For this review, take the finished solid that the model builds, in its own axes (mm). A direction names the side the tool comes from. Coordinates: 2 decimals unless noted, no trailing zeros. Order: outer loops, then holes, each group sorted by start corner. A loop starts at its lowest first (then second) coordinate and runs counter-clockwise, first axis right, second up.
from build123d import *

# Parameters (mm, degrees)
ESQUISSE1_W          = 50
ESQUISSE1_H          = 30
BASE_EXTRUSION_DEPTH = 10
PER_AGE1_D           = 5
PER_AGE1_CSINK_D     = 11
PER_AGE1_CSINK_ANGLE = 90
PER_AGE2_D           = 6
PER_AGE2_CBORE_D     = 11
PER_AGE2_CBORE_DEPTH = 6
CHANFREIN1_SIZE      = 5


with BuildPart() as part:
    # Esquisse1 → Base-Extrusion (new body)
    with BuildSketch(Plane.XY):
        with Locations((0, 15)):
            Rectangle(ESQUISSE1_W, ESQUISSE1_H)
    extrude(amount=BASE_EXTRUSION_DEPTH)

    # Perçage1 (through all)
    with Locations(Plane.XY.offset(10)):
        with Locations((15, 7.5)):
            per_age1 = CounterSinkHole(PER_AGE1_D / 2, PER_AGE1_CSINK_D / 2, counter_sink_angle=PER_AGE1_CSINK_ANGLE)

    # Symétrie1: Perçage1 across plane
    add(per_age1.mirror(Plane(origin=(0, 0, 0), x_dir=(0, 0, 1), z_dir=(1, 0, 0))), mode=Mode.SUBTRACT)

    # Perçage2 (through all)
    with Locations(Plane(origin=(0, 0, 0), x_dir=(-1, 0, 0), z_dir=(0, 0, -1))):
        with Locations((-15, 22.5)):
            per_age2 = CounterBoreHole(PER_AGE2_D / 2, PER_AGE2_CBORE_D / 2, PER_AGE2_CBORE_DEPTH)

    # Symétrie2: Perçage2 across plane
    add(per_age2.mirror(Plane(origin=(0, 0, 0), x_dir=(0, 0, 1), z_dir=(1, 0, 0))), mode=Mode.SUBTRACT)

    # Chanfrein1
    chanfrein1_edges = [part.edges().sort_by_distance(p)[0] for p in [
        (-25, 0, 5),
        (25, 0, 5),
    ]]
    chamfer(chanfrein1_edges, length=CHANFREIN1_SIZE)


solid = part.part
1. Take a section at A-A, the plane y = 7.5. Give the boundary of the cut face in (x, z).
Answer below:
outline: (-25, 0) - (-17.5, 0) - (-17.5, 7) - (-20.5, 10) - (-25, 10) - close; (-12.5, 0) - (12.5, 0) - (12.5, 7) - (9.5, 10) - (-9.5, 10) - (-12.5, 7) - close; (17.5, 0) - (25, 0) - (25, 10) - (20.5, 10) - (17.5, 7) - close
2. To check wall thickness, follow L1, parallel to Y at x = 15, z = 3.5; L2, parallel to X at y = 7.5, z = 4; L3, parallel to Y at x = -14, z = 8.5. State the ranges of each line that lie inside material, in increasing order.
Answer below:
L1: y = 0 to 5, 10 to 17, 28 to 30
L2: x = -25 to -17.5, -12.5 to 12.5, 17.5 to 25
L3: y = 0 to 3.63, 11.37 to 19.67, 25.33 to 30
3. Take a section at B-B, the plane x = -15. Give the boundary of the cut face in (y, z).
Answer below:
outline: (0, 0) - (5, 0) - (5, 7) - (2, 10) - (0, 10) - close; (10, 0) - (17, 0) - (17, 6) - (19.5, 6) - (19.5, 10) - (13, 10) - (10, 7) - close; (25.5, 6) - (28, 6) - (28, 0) - (30, 0) - (30, 10) - (25.5, 10) - close
4. Machinability: for faces 1 (the face through (-12, 22.6, 8)), 2 (the face through (15.716, 27.953, 2.958)), which of the approach directions +Z, -Z, +X, -X, +Y, -Y give a long, thin tool a straight path to every point of the face, cutting with its end or side? Answer none if there is none.
Answer below:
face 1: +Z, -Z
face 2: -Z
5. Clearance check with flat-ended pins moving along their axes: pin 1 Ø3.5 at (x, y) = (-15, 22.5) entering from -Z; pin 2 Ø8 at (x, y) = (15, 22.5) entering from -Z. State where each tip first meets the part, or that it passes through.
Answer below:
pin 1: passes through
pin 2: stops at z = 6
6. Take a section at C-C, the plane y = 22.5. Give the boundary of the cut face in (x, z), plus the area to 3 significant figures.
Answer below:
outline: (-25, 0) - (-20.5, 0) - (-20.5, 6) - (-18, 6) - (-18, 10) - (-25, 10) - close; (-12, 6) - (-9.5, 6) - (-9.5, 0) - (9.5, 0) - (9.5, 6) - (12, 6) - (12, 10) - (-12, 10) - close; (18, 6) - (20.5, 6) - (20.5, 0) - (25, 0) - (25, 10) - (18, 10) - close
area: 320 mm2
7. Take a section at D-D, the plane x = 16. Give the number of separate pieces and of enclosed holes in the cut face, plus the area to 3 significant figures.
Answer below:
separate pieces: 3
enclosed holes: 0
area: 157 mm2
8. The part is to be moulded in two halves that separate along X. For faces 3 (the face through (-25, 17, 5)), 4 (the face through (-13, 20, 6)), 5 (the face through (23, 3, 5)), say which applies: +X half, -X half, draft (parallel to the pull), parting line (faces both ways), or undercut.
Answer below:
face 3: -X half
face 4: undercut
face 5: +X half
